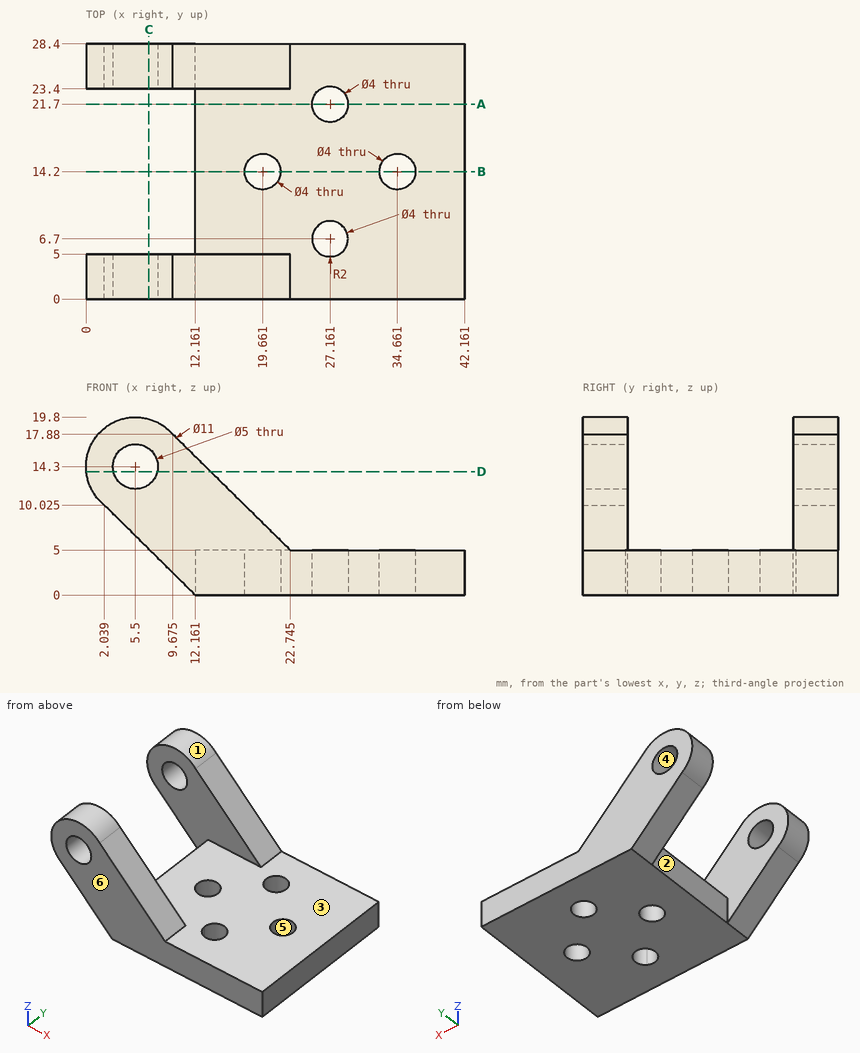
Here's the drawing with two shaded views (mm, measured from the low corner). I have some questions. A direction names the side the tool comes from. Coordinates: 2 decimals unless noted, no trailing zeros. Write each loop counter-clockwise with the first axis right and the second up, starting at its lowest first coordinate (ties: lowest second). Pieces come first, ordered by that corner, then holes. Notation, with made-up numbers: M 28,-2 L 33,-2 A21 cw 33,26 Z; hole C 42.25,-19 d11. An arc over 180 degrees is marked long. Write item = value, one per line. Start each with the question number.
Q1. If we section it at C-C, the plane x = 7: Write out the boundary of the cut face in (y, z).
Q2. If we section it at A-A, the plane y = 21.7: Write out the boundary of the cut face in (x, z), then the cut area to 3 significant figures.
Q3. On a 3-axis mill with a long thin cutter (end or side, diameter ignored), from which of +Z, -Z, +X, -X, +Y, -Y can I reach the whole of each face in a straight line? I mean the marked faces 1, 2 and 3. Say none if no direction works.
Q4. If we section it at B-B, the plane y = 14.2: Write out the boundary of the cut face in (x, z), then the cut area to 3 significant figures.
Q5. If we section it at D-D, the plane z = 13.75: Write out the boundary of the cut face in (x, y).
Q6. Thinking about a two-plate mould opening in Y: for the marked faces 4, 5 and 6, which applies, released by +Y, released by -Y, zero draft, split by the parting line, or undercut?
Q7. If I drill on L1, parallel to Y at x = 8, z = 8.25; L2, parallel to X at y = 14, z = 3; L3, parallel to X at y = 12.5, z = 2.5 (1 decimal), over which ranges is the centre line in solid material (lowest first)? Write a range as [from, to].
Q8. I'm going to push flat-ended pins straight in: pin 1 (1.5 mm diameter, centred on y = 3, z = 8.5, fed in from +X) (1 decimal); pin 2 (8.5 mm diameter, centred on x = 33.5, y = 20.5, fed in from +Z); pin 3 (1 mm diameter, centred on x = 11.5, y = 17.5, fed in from -Z); pin 4 (1.5 mm diameter, centred on y = 10.5, z = 2.5, fed in from -X). Where does each tip first touch, or does it pass through?
Check sheet entries:
q1.outline = M 0,5.11 L 5,5.11 L 5,12.3 L 0,12.3 Z; M 0,16.3 L 5,16.3 L 5,19.59 L 0,19.59 Z; M 23.4,5.11 L 28.4,5.11 L 28.4,12.3 L 23.4,12.3 Z; M 23.4,16.3 L 28.4,16.3 L 28.4,19.59 L 23.4,19.59 Z
q2.outline = M 12.16,0 L 25.16,0 L 25.16,5 L 12.16,5 Z; M 29.16,0 L 42.16,0 L 42.16,5 L 29.16,5 Z
q2.area = 130 mm²
q3.face_1 = +Y, -Y
q3.face_2 = +Z, -Z, -X
q3.face_3 = +Z, +X
q4.outline = M 12.16,0 L 17.66,0 L 17.66,5 L 12.16,5 Z; M 21.66,0 L 32.66,0 L 32.66,5 L 21.66,5 Z; M 36.66,0 L 42.16,0 L 42.16,5 L 36.66,5 Z
q4.area = 110 mm²
q5.outline = M 0.03,0 L 3.06,0 L 3.06,5 L 0.03,5 Z; M 0.03,23.4 L 3.06,23.4 L 3.06,28.4 L 0.03,28.4 Z; M 7.94,0 L 13.87,0 L 13.87,5 L 7.94,5 Z; M 7.94,23.4 L 13.87,23.4 L 13.87,28.4 L 7.94,28.4 Z
q6.face_4 = zero draft
q6.face_5 = undercut
q6.face_6 = released by -Y
q7.L1 = [0, 5], [23.4, 28.4]
q7.L2 = [12.16, 17.67], [21.65, 32.67], [36.65, 42.16]
q7.L3 = [12.2, 18.6], [20.7, 33.6], [35.7, 42.2]
q8.pin_1 = 20
q8.pin_2 = 5
q8.pin_3 = through
q8.pin_4 = 12.16
